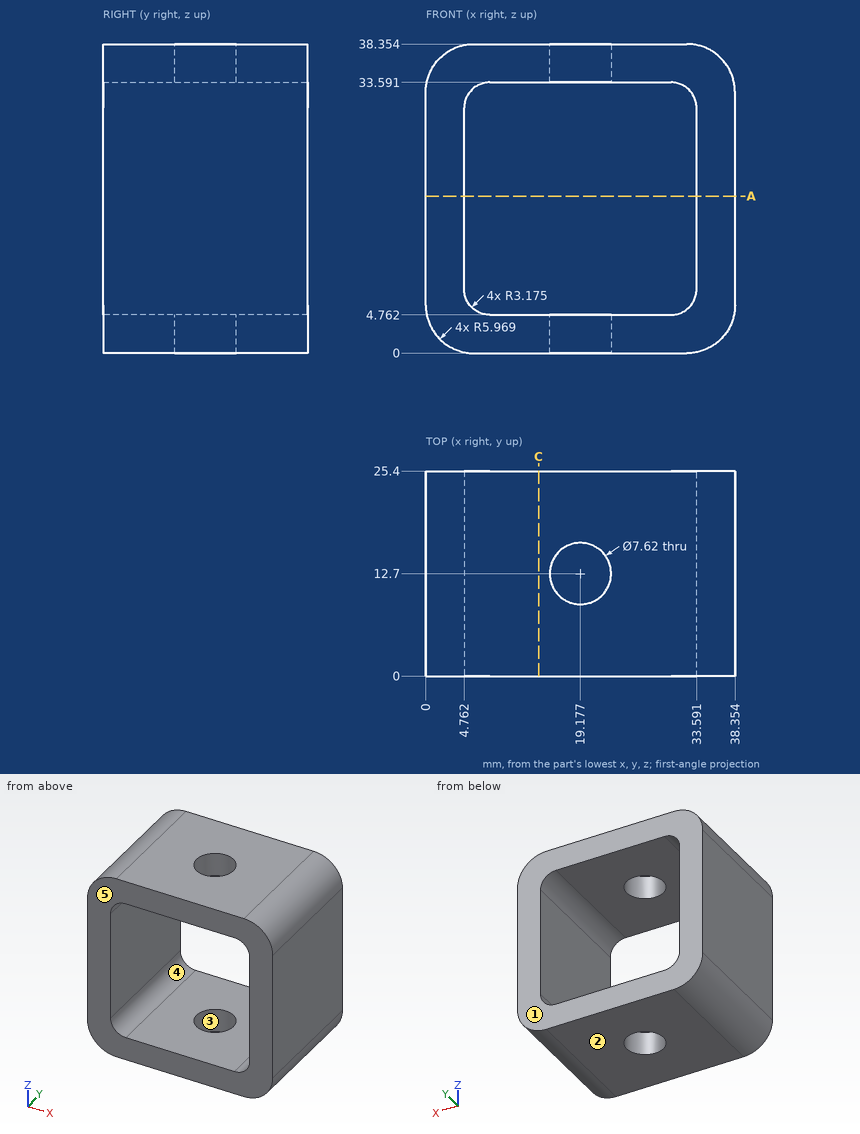
Part print with two shaded views. Sizes in mm from the minimum x, y, z corner. A direction names the side the tool comes from. Give positions to 0.01 mm unless a question says otherwise; leave off trailing zeros. Order: outer loops, then holes, each group sorted by start corner. A loop starts at its lowest first (then second) coordinate and runs counter-clockwise, first axis right, second up. Notation, with made-up numbers: M -4.75,77.25 L 9.25,77.25 A17 ccw 9.25,95.25 Z; hole C 10,-21 d9. An arc over 180 degrees is marked long. Put each result on its own line as item: value.
Item 1: Cut at C-C on x = 14. Write the cut outline in (y, z) (1 decimal).
Results are:
outline: M 0,0 L 25.4,0 L 25.4,4.8 L 0,4.8 Z; M 0,33.6 L 25.4,33.6 L 25.4,38.4 L 0,38.4 Z
Item 2: Pull direction Y, two halves, no side cores. Call the marked faces 1, 2 and 3: +Y half, -Y half, draft (parallel to the pull), parting line (faces both ways), or undercut.
Results are:
face 1: +Y half
face 2: draft
face 3: undercut
Item 3: Which spindle directions (+Z, -Z, +X, -X, +Y, -Y) get a long thin tool onto all of the face, cutting with end or side? Do the marked faces 4 and 5. Say none if no direction does.
Results are:
face 4: +Y, -Y
face 5: +Z, -Z, +X, -X, -Y
Item 4: Drop a flat-ended pin along its axis: pin 1 Ø10 at (x, z) = (21.5, 13.5) entering from +Y. Give the stop position or say it passes through.
Results are:
pin 1: through
Item 5: Wall check: probe 1 along X at (y, z) = (14.5, 23.5) (1 decimal); probe 2 along Z at (x, y) = (31.5, 11.75) (1 decimal). Give the ranges that are in metal, low to high.
Results are:
probe 1: 0 to 4.8, 33.6 to 38.4
probe 2: 0 to 5, 33.4 to 38.4
Item 6: Cut at A-A on z = 19.5. Write the cut outline in (x, y) (1 decimal).
Results are:
outline: M 0,0 L 4.8,0 L 4.8,25.4 L 0,25.4 Z; M 33.6,0 L 38.4,0 L 38.4,25.4 L 33.6,25.4 Z
